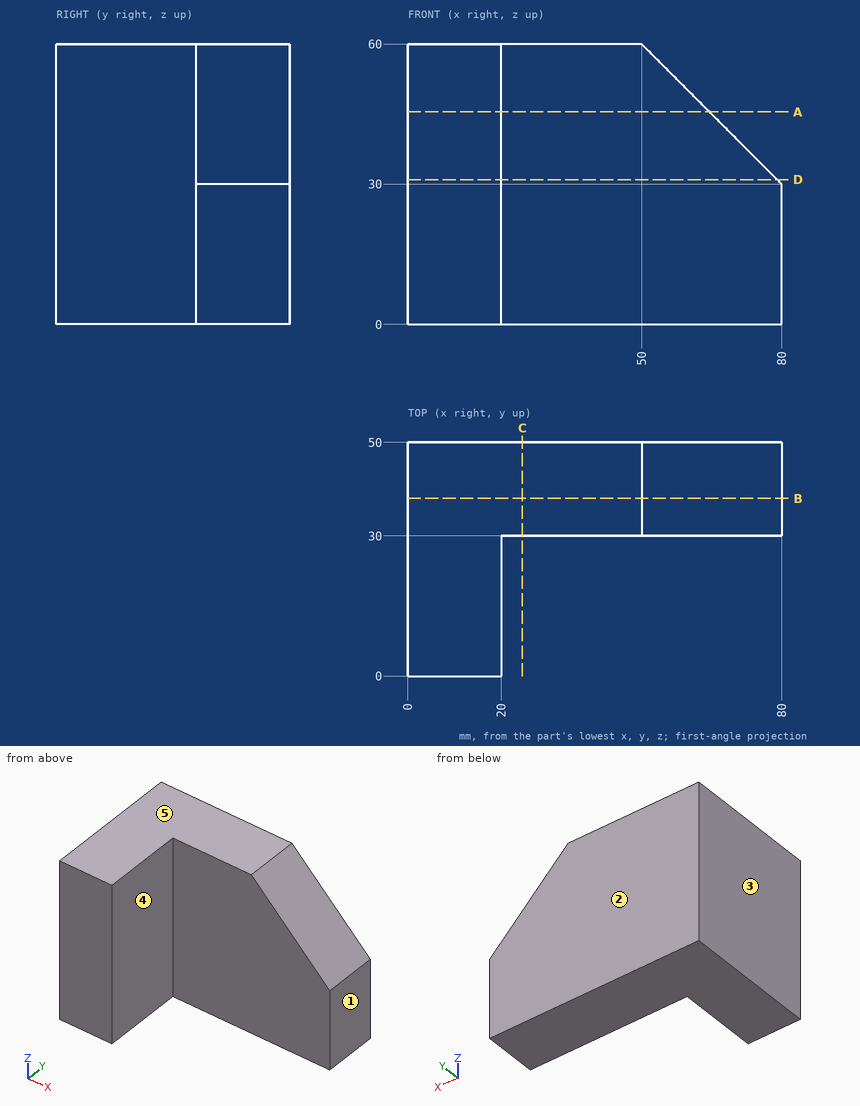
Geometry: see drawing. Coordinates: mm, zero at the bounding-box minimum. A direction names the side the tool comes from. Give positions to 0.01 mm unless a question says otherwise; leave off trailing zeros. Write each loop counter-clockwise with the first axis right and the second up, starting at its lowest first coordinate (ties: lowest second). Pieces come first, ordered by that corner, then holes. Notation, with made-up numbers: (51.5, -10) -> (96.5, -10) arc R26 ccw to (96.5, 16) -> close; hole circle Ø2 at (54, 1.25). An arc over 180 degrees is marked (long way). Use one line per item in the form item = value. Start each with the question number.
1) Ray query, probe 1 along X at (y, z) = (19.5, 19); probe 2 along Y at (x, z) = (64.5, 39.5); probe 3 along X at (y, z) = (40.5, 41). Return the intervals inside material, ascending. Write a range as from..to.
2) Draft query along X for the marked faces 1, 2 and 3. Return one class per face: pulls with the +X half, pulls with the -X half, needs draft (parallel to the pull), parting line crosses it, or undercut.
3) Section query A-A on z = 45.5. Return the cut outline in (x, y).
4) Pin query (flat end, axial travel): pin 1 (1.5 mm diameter, centred on x = 23.5, z = 13.5, fed in from -Y); pin 2 (4 mm diameter, centred on y = 27.5, z = 44, fed in from +X); pin 3 (5 mm diameter, centred on y = 33, z = 50.5, fed in from +X); pin 4 (1.5 mm diameter, centred on x = 58, y = 28, fed in from +Z). Return the tip coordinate at first contact, or that it passes through.
5) Section query C-C on x = 24.5. Return the cut outline in (y, z), then the cut area to 3 significant figures.
6) Section query D-D on z = 31. Return the cut outline in (x, y), then the cut area to 3 significant figures.
7) Section query B-B on y = 38. Return the cut outline in (x, z), then the cut area to 3 significant figures.
8) Set-up query: the marked faces 4 and 5. Return all of +Z, -Z, +X, -X, +Y, -Y with unobstructed straight access to the full face (end or side cutting, diameter ignored); none if empty.
Outcome:
q1.probe_1 = 0..20
q1.probe_2 = 30..50
q1.probe_3 = 0..69
q2.face_1 = pulls with the +X half
q2.face_2 = needs draft
q2.face_3 = pulls with the -X half
q3.outline = (0, 0) -> (20, 0) -> (20, 30) -> (64.5, 30) -> (64.5, 50) -> (0, 50) -> close
q4.pin_1 = 30
q4.pin_2 = 20
q4.pin_3 = 62
q4.pin_4 = through
q5.outline = (30, 0) -> (50, 0) -> (50, 60) -> (30, 60) -> close
q5.area = 1,200 mm^2
q6.outline = (0, 0) -> (20, 0) -> (20, 30) -> (79, 30) -> (79, 50) -> (0, 50) -> close
q6.area = 2,180 mm^2
q7.outline = (0, 0) -> (80, 0) -> (80, 30) -> (50, 60) -> (0, 60) -> close
q7.area = 4,350 mm^2
q8.face_4 = +Z, -Z, +X, -Y
q8.face_5 = +Z, +X, -X, +Y, -Y
